from build123d import *

# Parameters (mm, degrees)
SKETCH1_W           = 20
SKETCH1_H           = 60
BOSS_EXTRUDE1_DEPTH = 5
FILLET1_R           = 10
SKETCH2_R           = 4.95
BOSS_EXTRUDE2_DEPTH = 11
SKETCH2_4_R         = 5.05
CUT_EXTRUDE1_DEPTH  = 5
SKETCH4_W           = 10
SKETCH4_H           = 10
CUT_EXTRUDE2_DEPTH  = 5
SKETCH5_R           = 6.95
BOSS_EXTRUDE3_DEPTH = 5.2


with BuildPart() as part:
    # Sketch1 → Boss-Extrude1 (new body)
    with BuildSketch(Plane(origin=(0, 0, 0), x_dir=(1, 0, 0), z_dir=(0, 1, 0))):
        with Locations((-13.333333333, -1.025641026)):
            Rectangle(SKETCH1_W, SKETCH1_H)
    extrude(amount=BOSS_EXTRUDE1_DEPTH)

    # Fillet1
    fillet1_edges = [part.edges().sort_by_distance(p)[0] for p in [
        (-23.333333333, 2.5, -28.974358974),
        (-3.333333333, 2.5, -28.974358974),
        (-23.333333333, 2.5, 31.025641026),
        (-3.333333333, 2.5, 31.025641026),
    ]]
    fillet(fillet1_edges, radius=FILLET1_R - 0.0001)  # a hair under: the kernel refuses the full size

    # Sketch2 → Boss-Extrude2 (add)
    with BuildSketch(Plane(origin=(0, 5, 0), x_dir=(1, 0, 0), z_dir=(0, 1, 0))):
        with Locations(Location((-13.333333333, -21.025641026, 0), (0, 0, 90))):
            Circle(SKETCH2_R)
    extrude(amount=BOSS_EXTRUDE2_DEPTH)

    # Sketch2<4> → Cut-Extrude1 (cut)
    with BuildSketch(Plane(origin=(0, 5, 0), x_dir=(1, 0, 0), z_dir=(0, 1, 0))):
        with Locations(Location((-13.333333333, 18.974358974, 0), (0, 0, 270))):
            Circle(SKETCH2_4_R)
    extrude(amount=-CUT_EXTRUDE1_DEPTH, mode=Mode.SUBTRACT)

    # Sketch4 → Cut-Extrude2 (cut)
    with BuildSketch(Plane(origin=(0, 5, 0), x_dir=(1, 0, 0), z_dir=(0, 1, 0))):
        with Locations((-13.333333333, -1.025641026)):
            Rectangle(SKETCH4_W, SKETCH4_H)
    extrude(amount=-CUT_EXTRUDE2_DEPTH, mode=Mode.SUBTRACT)

    # Sketch5 → Boss-Extrude3 (add)
    with BuildSketch(Plane(origin=(0, 5, 0), x_dir=(1, 0, 0), z_dir=(0, 1, 0))):
        with Locations(Location((-13.333333333, -21.025641026, 0), (0, 0, 90))):
            Circle(SKETCH5_R)
    extrude(amount=BOSS_EXTRUDE3_DEPTH)


solid = part.part
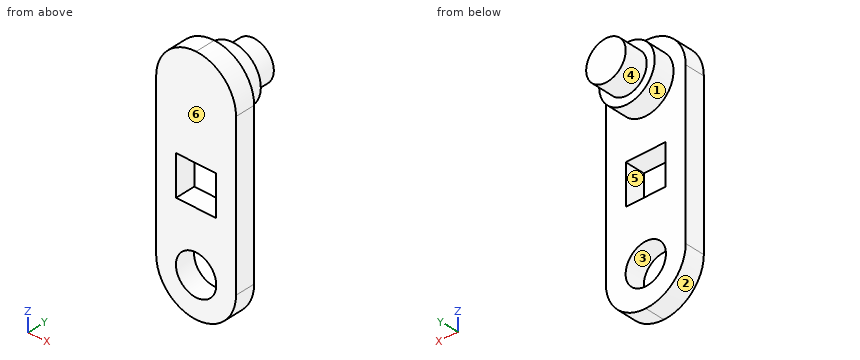
Could you check a few things on this model? Use its own coordinates, in mm. Face numbers are marked on the shaded views. A direction names the side the tool comes from. Coordinates: 2 decimals unless noted, no trailing zeros. Loops run counter-clockwise (first coordinate to the right, second up) from the corner with the lowest first, then second, coordinate; pieces in that order, holes last.
1. For the marked faces 4, 5 and 6, which set-ups out of +Z, -Z, +X, -X, +Y, -Y let a thin tool reach every point of the face, with its end or its side?
2. Imagine slicing it at C-C (y = 1.5). Give the number of separate pieces and of enclosed holes in the cut face, and give its area (3 significant figures).
3. We'd pull the mould along X, two halves only. Please class the marked faces 1, 2 and 3: released by +X, released by -X, zero draft, split by the parting line, or undercut.
4. Imagine slicing it at B-B (x = -16.5). Please give me the cut outline in (y, z).
5. Imagine slicing it at A-A (z = 5). Please give me the cut outline in (x, y), and give its area (3 significant figures).
6. For P1, Ø1.5, axis at x = -11, y = 5.5, coming from the -Z side; P2, Ø6, axis at x = -9, z = 3.5, coming from the +Y side; P3, Ø1.5, axis at x = -11.5, y = 3, coming from the +Z side, each with a flat end and sliding along its axis, tell me the tip position at first contact or that it passes through.
7. Imagine slicing it at D-D (z = -13). Please give me the cut outline in (x, y), and give its area (3 significant figures).
8. I need wall thicknesses on L1, parallel to X at y = 1.5, z = -2; L2, parallel to Z at x = -15.5, y = 3.5; L3, parallel to Z at x = -12, y = 3.75. Which ranges of each line are inside material? Lowest first, please.
Computed values:
1. face 4: +Y
1. face 5: +Y, -Y
1. face 6: +Z, -Z, +X, -X, -Y
2. separate pieces: 1
2. enclosed holes: 2
2. area: 934 mm2
3. face 1: split by the parting line
3. face 2: released by -X
3. face 3: undercut
4. outline: (0, -28.46) - (5, -28.46) - (5, -22.91) - (0, -22.91) - close; (0, -15.04) - (5, -15.04) - (5, -3.97) - (0, -3.97) - close; (0, 6.03) - (5, 6.03) - (5, 14.84) - (10.2, 14.84) - (10.2, 17.22) - (16, 17.22) - (16, 24.83) - (10.2, 24.83) - (10.2, 27.21) - (5, 27.21) - (5, 30.51) - (0, 30.51) - close
5. outline: (-23.33, 0) - (-18.33, 0) - (-18.33, 5) - (-23.33, 5) - close; (-8.33, 0) - (-3.33, 0) - (-3.33, 5) - (-8.33, 5) - close
5. area: 50.0 mm2
6. P1: stops at z = -28.82
6. P2: stops at y = 5
6. P3: stops at z = 30.97
7. outline: (-23.33, 0) - (-3.33, 0) - (-3.33, 5) - (-23.33, 5) - close
7. area: 100 mm2
8. L1: x = -23.33 to -18.33, -8.33 to -3.33
8. L2: z = -28.74 to -23.54, -14.41 to -3.97, 6.03 to 30.79
8. L3: z = -28.89 to -23.85, -14.1 to -3.97, 6.03 to 30.94
